from build123d import *

# Parameters (mm, degrees)
F0_W     = 15.113
F0_H     = 15.113
F1_DEPTH = 7.5565
F3_D     = 3.3274
F3_DEPTH = 12.7
F3_TIP   = 0.9996518119
F5_D     = 3.3274
F5_DEPTH = 12.7
F5_TIP   = 0.9996518119
F7_D     = 3.3274
F7_DEPTH = 12.7
F7_TIP   = 0.9996518119


with BuildPart() as f1:
    # F0 (on Front) → F1 (new body, symmetric)
    with BuildSketch(Plane.XZ):
        Rectangle(F0_W, F0_H)
    extrude(amount=F1_DEPTH, both=True)

    # F3
    with Locations(Plane.XZ.offset(7.5565)):
        with Locations((0, 0)):
            Hole(F3_D / 2, depth=F3_DEPTH)
            with Locations((0, 0, -(F3_DEPTH + F3_TIP / 2))):  # 118° drill point
                Cone(0, F3_D / 2, F3_TIP, mode=Mode.SUBTRACT)

    # F5
    with Locations(Plane.XY.offset(7.5565)):
        with Locations((0, 0)):
            Hole(F5_D / 2, depth=F5_DEPTH)
            with Locations((0, 0, -(F5_DEPTH + F5_TIP / 2))):  # 118° drill point
                Cone(0, F5_D / 2, F5_TIP, mode=Mode.SUBTRACT)

    # F7
    with Locations(Plane.YZ.offset(7.5565)):
        with Locations((0, 0)):
            Hole(F7_D / 2, depth=F7_DEPTH)
            with Locations((0, 0, -(F7_DEPTH + F7_TIP / 2))):  # 118° drill point
                Cone(0, F7_D / 2, F7_TIP, mode=Mode.SUBTRACT)


solid = f1.part
Could you check a few things on this model? Use its own coordinates, in mm. A direction names the side the tool comes from. Give positions to 0.01 mm unless a question says otherwise; leave off trailing zeros. Order: outer loops, then holes, each group sorted by start corner. A loop starts at its lowest first (then second) coordinate and runs counter-clockwise, first axis right, second up.
1. I need wall thicknesses on L1, parallel to X at y = 0, z = 6.25. Which ranges of the line are inside material? Lowest first, please.
Answers below:
L1: x = -7.56 to -1.66, 1.66 to 7.56
2. Suppose I cut it at A-A (y = -3). Write out the boundary of the cut face in (x, z).
Answers below:
outline: (-7.56, -7.56) - (7.56, -7.56) - (7.56, 7.56) - (-7.56, 7.56) - close; hole circle Ø3.33 at (0, 0)
3. For pin 1 (2.5 mm diameter, centred on y = 0, z = 0, fed in from +X); pin 2 (2.5 mm diameter, centred on x = 0, z = 0, fed in from -Y); pin 3 (3 mm diameter, centred on x = 0, y = 0, fed in from +Z), each with a flat end and sliding along its axis, tell me the tip position at first contact or that it passes through.
Answers below:
pin 1: stops at x = -5.39
pin 2: stops at y = 5.39
pin 3: stops at z = -5.24
4. Thinking about a two-plate mould opening in Y: for faces 1 (the flat face through (0, 7.556, 0)), 2 (the flat face through (0, 0, -7.556)), 3 (the cylindrical face through (1.662, 0.073, 4.322)), which applies, +Y half, -Y half, draft (parallel to the pull), parting line (faces both ways), or undercut?
Answers below:
face 1: +Y half
face 2: draft
face 3: undercut
5. Which directions (+Z, -Z, +X, -X, +Y, -Y) give clear straight access to the entire face, cutting with the end or side of a thin tool? Please do faces 4 (the cylindrical face through (-3.19, 1.23, 1.12)), 5 (the cylindrical face through (1.23, 1.12, -3.19)), 6 (the cylindrical face through (1.662, -4.322, 0.073)), 7 (the flat face through (-2, -7.556, 0)).
Answers below:
face 4: +X
face 5: +Z
face 6: -Y
face 7: +Z, -Z, +X, -X, -Y
